Work out the finished part from the listing and answer in its coordinate system (mm). A direction names the side the tool comes from. Coordinates: 2 decimals unless noted, no trailing zeros. Order: outer loops, then holes, each group sorted by start corner. A loop starts at its lowest first (then second) coordinate and runs counter-clockwise, first axis right, second up. Notation, with made-up numbers: M -22.75,68.5 L 3.25,68.5 A19 ccw 3.25,91.5 Z; hole C -24.75,50 d10. An arc over 180 degrees is marked long. Use a Markdown table: item, result.
from build123d import *

# Parameters (mm, degrees)
SKETCH1_R           = 8.75
BOSS_EXTRUDE1_DEPTH = 8.2
FILLET1_R           = 6
BOSS_EXTRUDE2_DEPTH = 9.4


with BuildPart() as part:
    # Sketch1 → Boss-Extrude1 (new body)
    with BuildSketch(Plane(origin=(0, 0, 0), x_dir=(1, 0, 0), z_dir=(0, 1, 0))):
        Circle(SKETCH1_R)
    extrude(amount=BOSS_EXTRUDE1_DEPTH)

    # Fillet1
    fillet1_edges = [part.edges().sort_by_distance(p)[0] for p in [
        (-8.75, 8.2, 0),
    ]]
    fillet(fillet1_edges, radius=FILLET1_R)

    # Sketch2 → Boss-Extrude2 (add)
    with BuildSketch(Plane.XZ):
        with BuildLine():
            ThreePointArc((4.292019342, -5.283154258), (6.146066324, -2.925579889), (6.806845742, 0))
            ThreePointArc((6.806845742, 0), (1.4e-08, 6.806845742), (-6.806845742, 2.9e-08))
            ThreePointArc((-6.806845742, 2.9e-08), (-6.146066331, -2.925579876), (-4.292019342, -5.283154258))
            Line((-4.292019342, -5.283154258), (4.292019342, -5.283154258))
        make_face()
    extrude(amount=BOSS_EXTRUDE2_DEPTH)


solid = part.part
(1) Given P1, Ø8, axis at y = 5.5, z = -4.5, coming from the +X side; P2, Ø5, axis at x = 1.5, y = 3.5, coming from the +Z side; P3, Ø3, axis at y = 5, z = 3.5, coming from the -X side; P4, Ø4.5, axis at x = -1.5, y = -4.5, coming from the -Z side, each flat-ended and moving along its own axis, determine where each tip first touches the part or whether it passes through.
Conclusion:
| item | result |
|---|---|
| P1 | x = 8.59 |
| P2 | z = 8.75 |
| P3 | x = -8.13 |
| P4 | z = -5.28 |
(2) Straight lines are drawn through the part: L1, parallel to Z at x = 0.25, y = -0.5; L2, parallel to X at y = 6.5, z = 4.75; L3, parallel to Z at x = 5.5, y = -3.75. For each, find the intervals that lie inside material, in ascending order.
Conclusion:
| item | result |
|---|---|
| L1 | -5.28 to 6.8 |
| L2 | -5.05 to 5.05 |
| L3 | -4.01 to 4.01 |
(3) A cutting plane is placed at A-A (y = -7.5). Determine the outline of the cut face in (x, z).
Conclusion:
| item | result |
|---|---|
| outline | M -4.29,-5.28 L 4.29,-5.28 A6.81 ccw long Z |
(4) Which of the six approach directions +Z, -Z, +X, -X, +Y, -Y give full straight-line access (tool end or side, diameter ignored) to faces 1 (the flat face through (0, -5, -5.283)), 2 (the flat face through (0, 0, -6)), 3 (the flat face through (0, 8.2, 0))?
Conclusion:
| item | result |
|---|---|
| face 1 | -Z, +X, -X, -Y |
| face 2 | -Y |
| face 3 | +Z, -Z, +X, -X, +Y |
